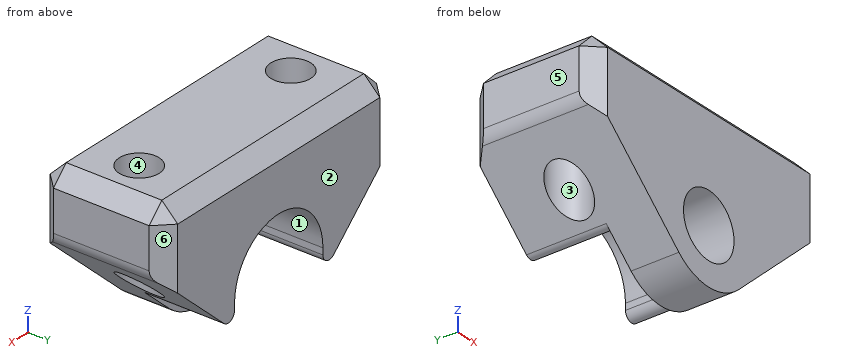
from build123d import *

# Parameters (mm, degrees)
SKETCH_1_R          = 2
EXTRUDE_1_DEPTH     = 4
HOLE_WIZARD_M3_1_D  = 2.5
CUT_EXTRUDE_1_DEPTH = 5
CHAMFER_1_SIZE      = 1
FILLET_1_R          = 1
FILLET_2_R          = 0.5


with BuildPart() as part:
    # 草图1 → 凸台-拉伸1 (new body, symmetric)
    with BuildSketch(Plane(origin=(0, 0, 0), x_dir=(1, 0, 0), z_dir=(0, 1, 0))):
        with BuildLine():
            Line((9, -7.5), (-9, -7.5))
            Line((-9, -7.5), (-9, -3.5))
            Line((-9, -3.5), (-2.36461126, 2.580428954))
            ThreePointArc((-2.36461126, 2.580428954), (0, 3.5), (2.36461126, 2.580428954))
            Line((2.36461126, 2.580428954), (9, -3.5))
            Line((9, -3.5), (9, -7.5))
        make_face()
        Circle(SKETCH_1_R, mode=Mode.SUBTRACT)
    extrude(amount=EXTRUDE_1_DEPTH, both=True)

    # M3 螺纹孔1 (through all)
    with Locations(Plane.XY.offset(7.5)):
        with Locations((-6, 0), (6, 0)):
            Hole(HOLE_WIZARD_M3_1_D / 2)

    # 草图4 → 切除-拉伸1 (cut)
    with BuildSketch(Plane(origin=(0, 4, 0), x_dir=(1, 0, 0), z_dir=(0, 1, 0))):
        with BuildLine():
            Line((-3.5, 0), (-3.5, 1.54))
            Line((-3.5, 1.54), (-2.36461126, 2.580428954))
            ThreePointArc((-2.36461126, 2.580428954), (0, 3.5), (2.36461126, 2.580428954))
            Line((2.36461126, 2.580428954), (3.5, 1.54))
            Line((3.5, 1.54), (3.5, 0))
            ThreePointArc((3.5, 0), (0, -3.5), (-3.5, 0))
        make_face()
    extrude(amount=-CUT_EXTRUDE_1_DEPTH, mode=Mode.SUBTRACT)

    # 倒角1
    chamfer_1_edges = [part.edges().sort_by_distance(p)[0] for p in [
        (9, 0, 7.5),
        (-9, 0, 7.5),
        (-9, 4, 5.5),
        (0, 4, 7.5),
        (9, 4, 5.5),
        (0, -4, 7.5),
        (-9, -4, 5.5),
        (9, -4, 5.5),
    ]]
    chamfer(chamfer_1_edges, length=CHAMFER_1_SIZE)

    # 圆角1
    fillet_1_edges = [part.edges().sort_by_distance(p)[0] for p in [
        (-9, 0, 3.5),
        (9, 0, 3.5),
    ]]
    fillet(fillet_1_edges, radius=FILLET_1_R)

    # 圆角2
    fillet_2_edges = [part.edges().sort_by_distance(p)[0] for p in [
        (-3.5, 1.5, -1.54),
        (3.5, 1.5, -1.54),
    ]]
    fillet(fillet_2_edges, radius=FILLET_2_R)


solid = part.part
The listing builds one solid part. Answer for the finished solid, in the listing's coordinates (mm). Face numbers are marked on the shaded views. A direction names the side the tool comes from. Give positions to 0.01 mm unless a question says otherwise; leave off trailing zeros. Write each loop counter-clockwise with the first axis right and the second up, starting at its lowest first coordinate (ties: lowest second). Pieces come first, ordered by that corner, then holes.
Item 1: Section C-C, the plane y = -2 is taken. Write down the section's boundary in (x, z), plus the area to 3 significant figures.
Item 2: Which of the six approach directions +Z, -Z, +X, -X, +Y, -Y give full straight-line access (tool end or side, diameter ignored) to the marked faces 1 and 2?
Item 3: Section B-B, the plane x = 0 is taken. Write down the section's boundary in (y, z), plus the area to 3 significant figures.
Item 4: Determine the mould class of the marked faces 3, 4, 5 and 6 for opening direction Y: released by +Y, released by -Y, zero draft, split by the parting line, or undercut.
Item 5: Find the intervals of material crossed by line 1 along X through (y, z) = (0, 5.25); line 2 along Y through (x, z) = (6, 5.75); line 3 along Z through (x, y) = (-4, 0.75), in increasing order.
Item 6: Section A-A, the plane z = 5.75 is taken. Write down the section's boundary in (x, y), plus the area to 3 significant figures.
Item 7: Flat-ended cylindrical pins translate along their axes: P1, Ø5.5, axis at x = 1, z = 1.5, coming from the +Y side; P2, Ø4, axis at y = -3, z = 1.5, coming from the +X side; P3, Ø2, axis at x = 6, y = 0, coming from the +Z side; P4, Ø4.5, axis at x = 0, z = 0, coming from the +Y side. Find the tip coordinate at first contact, or state that the pin passes through.
Item 8: Section D-D, the plane y = -0.25 is taken. Write down the section's boundary in (x, z), plus the area to 3 significant figures.
Completed:
1. outline: (-9, 3.94) arc R1 ccw to (-8.68, 3.2) - (-2.36, -2.58) arc R3.5 ccw to (2.36, -2.58) - (8.68, 3.2) arc R1 ccw to (9, 3.94) - (9, 6.5) - (8, 7.5) - (-8, 7.5) - (-9, 6.5) - close; hole circle Ø4 at (0, 0)
1. area: 130 mm2
2. face 1: -Z, +Y
2. face 2: +Z, -Z, +X, -X, +Y
3. outline: (-4, -3.5) - (-1, -3.5) - (-1, -2) - (-4, -2) - close; (-4, 2) - (-1, 2) - (-1, 3.5) - (4, 3.5) - (4, 6.5) - (3, 7.5) - (-3, 7.5) - (-4, 6.5) - close
3. area: 40.0 mm2
4. face 3: undercut
4. face 4: undercut
4. face 5: zero draft
4. face 6: released by +Y
5. line 1: x = -9 to -7.25, -4.75 to 4.75, 7.25 to 9
5. line 2: y = -4 to -1.25, 1.25 to 4
5. line 3: z = -0.9 to 7.5
6. outline: (-9, -3) - (-8, -4) - (8, -4) - (9, -3) - (9, 3) - (8, 4) - (-8, 4) - (-9, 3) - close; hole circle Ø2.5 at (-6, 0); hole circle Ø2.5 at (6, 0)
6. area: 132 mm2
7. P1: stops at y = 4
7. P2: stops at x = 8.9
7. P3: passes through
7. P4: stops at y = -1
8. outline: (-9, 3.94) arc R1 ccw to (-8.68, 3.2) - (-7.22, 1.87) - (-7.22, 7.5) - (-8, 7.5) - (-9, 6.5) - close; (-4.78, -0.37) - (-4.34, -0.77) arc R0.5 ccw to (-3.5, -0.4) - (-3.5, 0) arc R3.5 cw to (3.5, 0) - (3.5, -0.4) arc R0.5 ccw to (4.34, -0.77) - (4.78, -0.37) - (4.78, 7.5) - (-4.78, 7.5) - close; (7.22, 1.87) - (8.68, 3.2) arc R1 ccw to (9, 3.94) - (9, 6.5) - (8, 7.5) - (7.22, 7.5) - close
8. area: 70.3 mm2
